from build123d import *

# Parameters (mm, degrees)
SKETCH_1_W          = 52
SKETCH_1_H          = 14
EXTRUDE_1_DEPTH     = 11
SHELL_1_T           = -2
SKETCH_2_W          = 24
SKETCH_2_H          = 10
CUT_EXTRUDE_1_DEPTH = 2
SKETCH_3_W          = 24
SKETCH_3_H          = 2
EXTRUDE_2_DEPTH     = 11
SKETCH_8_R          = 2
CUT_EXTRUDE_5_DEPTH = 2
FILLET_1_R          = 1
SKETCH_15_W         = 4
SKETCH_15_H         = 4
EXTRUDE_4_DEPTH     = 3
SKETCH_16_R         = 0.8
CUT_EXTRUDE_7_DEPTH = 3
SKETCH_17_W         = 24
SKETCH_17_H         = 10
CUT_EXTRUDE_8_DEPTH = 0.4


with BuildPart() as part:
    # 草图1 → 凸台-拉伸1 (new body)
    with BuildSketch(Plane.XY):
        with Locations((26, 7)):
            Rectangle(SKETCH_1_W, SKETCH_1_H)
    extrude(amount=EXTRUDE_1_DEPTH)

    # 抽壳1
    shell_1_openings = [part.faces().sort_by_distance(p)[0] for p in [
        (26, 7, 0),
    ]]
    offset(amount=SHELL_1_T, openings=shell_1_openings, kind=Kind.INTERSECTION)

    # 草图2 → 切除-拉伸1 (cut)
    with BuildSketch(Plane(origin=(0, 0, 9), x_dir=(-1, 0, 0), z_dir=(0, 0, -1))):
        with Locations((-26, 7)):
            Rectangle(SKETCH_2_W, SKETCH_2_H)
    extrude(amount=-CUT_EXTRUDE_1_DEPTH, mode=Mode.SUBTRACT)

    # 草图3 → 凸台-拉伸2 (add)
    with BuildSketch(Plane.XY.offset(11)):
        with Locations((26, 1)):
            Rectangle(SKETCH_3_W, SKETCH_3_H)
        with Locations((26, 13)):
            Rectangle(SKETCH_3_W, SKETCH_3_H)
    extrude(amount=EXTRUDE_2_DEPTH)

    # 草图8 → 切除-拉伸5 (cut)
    with BuildSketch(Plane.XY.offset(11)):
        with Locations((8, 7)):
            Circle(SKETCH_8_R)
        with Locations((44, 7)):
            Circle(SKETCH_8_R)
    extrude(amount=-CUT_EXTRUDE_5_DEPTH, mode=Mode.SUBTRACT)

    # 圆角1
    fillet_1_edges = [part.edges().sort_by_distance(p)[0] for p in [
        (45, 14, 11),
        (45, 0, 11),
        (7, 14, 11),
        (38, 0, 16.5),
        (14, 0, 16.5),
        (0, 7, 11),
        (26, 14, 0),
        (14, 14, 16.5),
        (38, 14, 16.5),
        (52, 7, 0),
        (26, 0, 0),
        (0, 7, 0),
        (0, 14, 5.5),
        (52, 14, 5.5),
        (52, 0, 5.5),
        (0, 0, 5.5),
        (7, 0, 11),
    ]]
    fillet(fillet_1_edges, radius=FILLET_1_R)

    # 草图15 → 凸台-拉伸4 (add)
    with BuildSketch(Plane.XY.offset(22)):
        with Locations((26, 4)):
            Rectangle(SKETCH_15_W, SKETCH_15_H)
        with Locations((26, 10)):
            Rectangle(SKETCH_15_W, SKETCH_15_H)
    extrude(amount=-EXTRUDE_4_DEPTH)

    # 草图16 → 切除-拉伸7 (cut)
    with BuildSketch(Plane.XY.offset(22)):
        with Locations((26, 10)):
            Circle(SKETCH_16_R)
        with Locations((26, 4)):
            Circle(SKETCH_16_R)
    extrude(amount=-CUT_EXTRUDE_7_DEPTH, mode=Mode.SUBTRACT)

    # 草图19 → 切除-旋转6 (revolve, cut)
    with BuildSketch(Plane(origin=(0, 7, 0), x_dir=(1, 0, 0), z_dir=(0, 1, 0)), mode=Mode.PRIVATE) as cut_revolve_6_sk:
        Polygon((2.1, -11), (3.5, -11), (3.5, -9), (2.7, -9), (2.7, -9.9), align=None)
    revolve(cut_revolve_6_sk.sketch.rotate(Axis((3.5, 7, 11), (0, 0, -1)), 270), axis=Axis((3.5, 7, 11), (0, 0, -1)), mode=Mode.SUBTRACT)

    # 草图20 → 切除-旋转7 (revolve, cut)
    with BuildSketch(Plane(origin=(0, 7, 0), x_dir=(1, 0, 0), z_dir=(0, 1, 0)), mode=Mode.PRIVATE) as cut_revolve_7_sk:
        Polygon((11.1, -11), (12.5, -11), (12.5, -9), (11.7, -9), (11.7, -9.9), align=None)
    revolve(cut_revolve_7_sk.sketch.rotate(Axis((12.5, 7, 11), (0, 0, -1)), 270), axis=Axis((12.5, 7, 11), (0, 0, -1)), mode=Mode.SUBTRACT)

    # 草图21 → 切除-旋转8 (revolve, cut)
    with BuildSketch(Plane(origin=(0, 7, 0), x_dir=(1, 0, 0), z_dir=(0, 1, 0)), mode=Mode.PRIVATE) as cut_revolve_8_sk:
        Polygon((38.1, -11), (39.5, -11), (39.5, -9), (38.7, -9), (38.7, -9.9), align=None)
    revolve(cut_revolve_8_sk.sketch.rotate(Axis((39.5, 7, 11), (0, 0, -1)), 270), axis=Axis((39.5, 7, 11), (0, 0, -1)), mode=Mode.SUBTRACT)

    # 草图22 → 切除-旋转9 (revolve, cut)
    with BuildSketch(Plane(origin=(0, 7, 0), x_dir=(1, 0, 0), z_dir=(0, 1, 0)), mode=Mode.PRIVATE) as cut_revolve_9_sk:
        Polygon((47.1, -11), (48.5, -11), (48.5, -9), (47.7, -9), (47.7, -9.9), align=None)
    revolve(cut_revolve_9_sk.sketch.rotate(Axis((48.5, 7, 11), (0, 0, -1)), 270), axis=Axis((48.5, 7, 11), (0, 0, -1)), mode=Mode.SUBTRACT)

    # 草图17 → 切除-拉伸8 (cut)
    with BuildSketch(Plane.XY.offset(22)):
        with Locations((26, 7)):
            Rectangle(SKETCH_17_W, SKETCH_17_H)
    extrude(amount=-CUT_EXTRUDE_8_DEPTH, mode=Mode.SUBTRACT)


solid = part.part
CAD build for the part. Positions are in the model's coordinates, mm. A direction names the side the tool comes from. Give positions to 0.01 mm unless a question says otherwise; leave off trailing zeros. Order: outer loops, then holes, each group sorted by start corner. A loop starts at its lowest first (then second) coordinate and runs counter-clockwise, first axis right, second up. Notation, with made-up numbers: (-27, 21) - (-10, 21) arc R27 cw to (-10, 58) - close; hole circle Ø8 at (19, -26). An arc over 180 degrees is marked (long way). Write each question's results on one line, items separated by ' | '.
1. Saw through at D-D on z = 3.75. List the corners of the cut face in (x, y), and give its area (3 significant figures).
Calculated:
outline: (0, 1) arc R1 ccw to (1, 0) - (51, 0) arc R1 ccw to (52, 1) - (52, 13) arc R1 ccw to (51, 14) - (1, 14) arc R1 ccw to (0, 13) - close; hole (2, 2) - (50, 2) - (50, 12) - (2, 12) - close | area: 247 mm2
2. Saw through at C-C on y = 10. List the corners of the cut face in (x, z), and give its area (3 significant figures).
Calculated:
outline: (0, 1) arc R1 ccw to (1, 0) - (2, 0) - (2, 9) - (14, 9) - (14, 11) - (1, 11) arc R1 ccw to (0, 10) - close; (24, 19) - (25.2, 19) - (25.2, 21.6) - (24, 21.6) - close; (26.8, 19) - (28, 19) - (28, 21.6) - (26.8, 21.6) - close; (38, 9) - (50, 9) - (50, 0) - (51, 0) arc R1 ccw to (52, 1) - (52, 11) - (38, 11) - close | area: 97.6 mm2
3. Saw through at A-A on z = 20.5. List the corners of the cut face in (x, y), and give its area (3 significant figures).
Calculated:
outline: (14, 1) arc R1 ccw to (15, 0) - (37, 0) arc R1 ccw to (38, 1) - (38, 2) - (28, 2) - (28, 6) - (24, 6) - (24, 2) - (14, 2) - close; (14, 12) - (24, 12) - (24, 8) - (28, 8) - (28, 12) - (38, 12) - (38, 13) arc R1 ccw to (37, 14) - (15, 14) arc R1 ccw to (14, 13) - close; hole circle Ø1.6 at (26, 4); hole circle Ø1.6 at (26, 10) | area: 123 mm2
4. Probe L1, parallel to Y at x = 26, z = 20.25; L2, parallel to Y at x = 20.5, z = 1; L3, parallel to Y at x = 39.5, z = 9.65. List the from-to ranges inside material, lowest first. Write a range as from..to.
Calculated:
L1: y = 0..3.2, 4.8..6, 8..9.2, 10.8..14 | L2: y = 0..2, 12..14 | L3: y = 0..6.2, 7.8..14
5. Saw through at B-B on x = 3.5. List the corners of the cut face in (y, z), and give its area (3 significant figures).
Calculated:
outline: (0, 1) arc R1 ccw to (1, 0) - (2, 0) - (2, 9) - (6.2, 9) - (6.2, 9.9) - (5.6, 11) - (1, 11) arc R1 ccw to (0, 10) - close; (7.8, 9) - (12, 9) - (12, 0) - (13, 0) arc R1 ccw to (14, 1) - (14, 10) arc R1 ccw to (13, 11) - (8.4, 11) - (7.8, 9.9) - close | area: 59.3 mm2
6. Pull direction Y, two halves, no side cores. Call faces 4 (the face through (0.301, 0.285, 5.563)), 5 (the face through (28, 10, 20)), 6 (the face through (14, 1.5, 16.4)), 7 (the face through (26, 2, 8)): released by +Y, released by -Y, zero draft, split by the parting line, or undercut.
Calculated:
face 4: released by -Y | face 5: undercut | face 6: zero draft | face 7: undercut
7. 3-axis set-ups, long thin cutter, end or side, ignore diameter. For faces 1 (the face through (25, 10, 19)), 2 (the face through (38, 1.5, 16.4)), 3 (the face through (6, 8, 11)): which of +Z, -Z, +X, -X, +Y, -Y reach the whole face in a straight line?
Calculated:
face 1: -Z, +X, -X | face 2: +Z, +X, +Y, -Y | face 3: +Z, -X, +Y, -Y
8. Pin check, flat tips, straight feed: pin 1 (1 mm diameter, centred on x = 39.5, y = 7, fed in from -Z); pin 2 (0.8 mm diameter, centred on y = 9.5, z = 20.5, fed in from +X); pin 3 (5 mm diameter, centred on x = 9, y = 5, fed in from -Z); pin 4 (3 mm diameter, centred on y = 3, z = 19.5, fed in from -X). Stop position of each tip, or through.
Calculated:
pin 1: passes through | pin 2: stops at x = 28 | pin 3: stops at z = 9 | pin 4: stops at x = 14
